Could you check a few things on this model? Use its own coordinates, in mm. Face numbers are marked on the shaded views. A direction names the side the tool comes from. Coordinates: 2 decimals unless noted, no trailing zeros. Order: outer loops, then holes, each group sorted by start corner. A loop starts at its lowest first (then second) coordinate and runs counter-clockwise, first axis right, second up. Notation, with made-up numbers: (-5, 47.25) - (2, 47.25) arc R29 ccw to (2, 75.25) - close; hole circle Ø7 at (80, 52.5). An arc over 180 degrees is marked (long way). One line per item, written item: value.
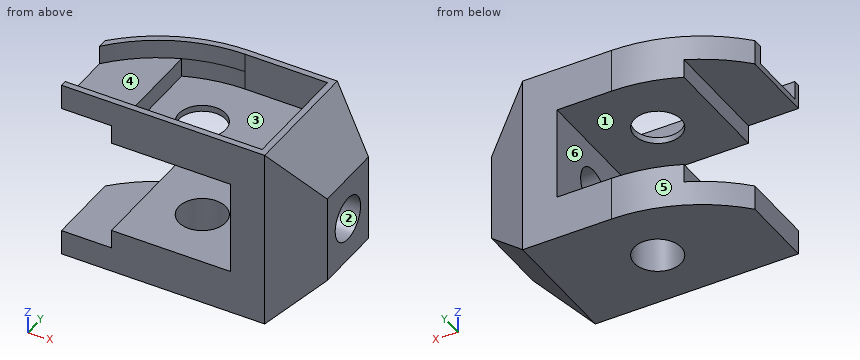
from build123d import *

# Parameters (mm, degrees)
SKETCH2_R           = 7.5
BOSS_EXTRUDE1_DEPTH = 29
CUT_EXTRUDE1_DEPTH  = 95.026591983
SKETCH4_R           = 7
CUT_EXTRUDE2_DEPTH  = 95.026591983
CUT_EXTRUDE5_DEPTH  = 6
CUT_EXTRUDE7_DEPTH  = 6


with BuildPart() as part:
    # Sketch2 → Boss-Extrude1 (new, symmetric)
    with BuildSketch(Plane.XY):
        with BuildLine():
            Line((0, 0), (0, 24))
            ThreePointArc((0, 24), (16.66060556, 35.82575695), (36.66060556, 40))
            Line((36.66060556, 40), (65, 40))
            Line((65, 40), (80, 31.339745962))
            Line((80, 31.339745962), (80, 8.660254038))
            Line((80, 8.660254038), (65, 0))
            Line((65, 0), (0, 0))
        make_face()
        with Locations(Location((34, 19, 0), (0, 0, 180))):
            Circle(SKETCH2_R, mode=Mode.SUBTRACT)
    extrude(amount=BOSS_EXTRUDE1_DEPTH, both=True)

    # Sketch3 → Cut-Extrude1 (cut, through all)
    with BuildSketch(Plane(origin=(0, 40, 0), x_dir=(1, 0, 0), z_dir=(0, 1, 0))):
        Polygon((65, 29), (80, 29), (80, 14), align=None)
        Polygon((0, 21), (16, 21), (16, 15), (54, 15), (54, -15), (16, -15), (16, -21), (0, -21), align=None)
        Polygon((80, -29), (80, -14), (65, -29), align=None)
    extrude(amount=-CUT_EXTRUDE1_DEPTH, mode=Mode.SUBTRACT)

    # Sketch4 → Cut-Extrude2 (cut, through all)
    with BuildSketch(Plane(origin=(80, 0, 0), x_dir=(0, 0, -1), z_dir=(1, 0, 0))):
        with Locations((0, 20)):
            Circle(SKETCH4_R)
    extrude(amount=-CUT_EXTRUDE2_DEPTH, mode=Mode.SUBTRACT)

    # Sketch5 → Cut-Extrude5 (cut)
    with BuildSketch(Plane.XY.offset(29)):
        with BuildLine():
            Line((0, 20.98386677), (0, 2))
            Line((0, 2), (63, 2))
            Line((63, 2), (63, 38))
            Line((63, 38), (36.66060556, 38))
            ThreePointArc((36.66060556, 38), (16.452013389, 33.538635744), (0, 20.98386677))
        make_face()
    extrude(amount=-CUT_EXTRUDE5_DEPTH, mode=Mode.SUBTRACT)

    # Sketch9 → Cut-Extrude7 (cut)
    with BuildSketch(Plane.XY.offset(23)):
        with BuildLine():
            Line((63, 2), (63, 38))
            Line((63, 38), (36.66060556, 38))
            ThreePointArc((36.66060556, 38), (27.381262347, 37.09451974), (18.452013389, 34.412241231))
            Line((18.452013389, 34.412241231), (18.452013389, 2))
            Line((18.452013389, 2), (63, 2))
        make_face()
    extrude(amount=-CUT_EXTRUDE7_DEPTH, mode=Mode.SUBTRACT)


solid = part.part
Item 1: I want a section at C-C on x = 28. Please give me the cut outline in (y, z), then the cut area to 3 significant figures.
Conclusion:
outline: (0, -29) - (14.5, -29) - (14.5, -15) - (0, -15) - close; (0, 15) - (14.5, 15) - (14.5, 17) - (2, 17) - (2, 29) - (0, 29) - close; (23.5, -29) - (39.24, -29) - (39.24, -15) - (23.5, -15) - close; (23.5, 15) - (39.24, 15) - (39.24, 29) - (37.21, 29) - (37.21, 17) - (23.5, 17) - close
area: 532 mm²
Item 2: For the marked faces 1, 2 and 3, which set-ups out of +Z, -Z, +X, -X, +Y, -Y let a thin tool reach every point of the face, with its end or its side?
Conclusion:
face 1: -X, +Y, -Y
face 2: +X, -X
face 3: +Z
Item 3: Thinking about a two-plate mould opening in Y: for the marked faces 4, 5 and 6, which applies, pulls with the +Y half, pulls with the -Y half, needs draft (parallel to the pull), parting line crosses it, or undercut?
Conclusion:
face 4: undercut
face 5: pulls with the +Y half
face 6: needs draft
Item 4: If I drill on probe 1 along Z at (x, y) = (49.5, 30.5); probe 2 along Z at (x, y) = (5, 21); probe 3 along X at (y, z) = (17.5, 22), over which ranges is the centre line in solid material (lowest first)?
Conclusion:
probe 1: -29 to -15, 15 to 17
probe 2: -29 to -21, 21 to 23
probe 3: 0 to 18.45, 63 to 72
Item 5: I want a section at D-D on y = 20. Give the number of separate pieces and of enclosed holes in the cut face, then the cut area to 3 significant figures.
Conclusion:
separate pieces: 4
enclosed holes: 0
area: 1,360 mm²
Item 6: I'm going to push flat-ended pins straight in: pin 1 Ø1.8 at (y, z) = (23.5, -17) entering from -X; pin 2 Ø3 at (x, y) = (39.5, 10.5) entering from +Z; pin 3 Ø9.5 at (x, z) = (20.5, 22.5) entering from +Y. Where does each tip first touch, or does it pass through?
Conclusion:
pin 1: x = 16
pin 2: z = 17
pin 3: y = 38.68
Item 7: I want a section at A-A on x = 56.5. Please give me the cut outline in (y, z), then the cut area to 3 significant figures.
Conclusion:
outline: (0, -29) - (40, -29) - (40, 29) - (38, 29) - (38, 17) - (2, 17) - (2, 29) - (0, 29) - close; hole circle Ø14 at (20, 0)
area: 1,730 mm²
Item 8: I want a section at B-B on z = 0. Please give me the cut outline in (x, y), then the cut area to 3 significant figures.
Conclusion:
outline: (54, 0) - (65, 0) - (80, 8.66) - (80, 13) - (54, 13) - close; (54, 27) - (80, 27) - (80, 31.34) - (65, 40) - (54, 40) - close
area: 546 mm²
